Autodesk Inventor part; units mm, degrees
ref_plane "YZ Plane" through (0, 0, 0) normal (1, 0, 0) x (0, 1, 0)
ref_plane "XZ Plane" through (0, 0, 0) normal (0, 1, 0) x (-1, 0, 0)
ref_plane "XY Plane" through (0, 0, 0) normal (0, 0, 1) x (1, 0, 0)
sketch "Sketch1" plane through (0, 0, 0) normal (0, 0, 1) x (1, 0, 0)
  line L0 (5.6444, -5.6444) -> (-5.6444, -5.6444)
  line L1 (-5.6444, -5.6444) -> (-5.6444, 5.6444)
  line L2 (-5.6444, 5.6444) -> (5.6444, 5.6444)
  line L3 (5.6444, 5.6444) -> (5.6444, -5.6444)
  point P0 (0, 0)
  point P1 (0, 0)
  dimension "d0" = 11.2889
extrude "Extrusion1" add sketch "Sketch1" along normal blind 8.4667
ref_plane "Work Plane1" through (0, 5.6444, 8.4667) normal (-1, 0, 0) x (0, -1, 0)
sketch "Sketch2" plane through (0, 5.6444, 8.4667) normal (-1, 0, 0) x (0, -1, 0)
  line L0 (5.6444, -8.4667) -> (-7.0556, -8.4667)
  line L1 (0, -8.4667) -> (11.2889, -8.4667)
  line L2 (5.6444, -8.4667) -> (5.6444, -14.8167)
  arc A0 (-7.0556, -8.4667) -> (5.6444, -14.8167) centre (5.6444, 1.0583) ccw
  dimension "d3" = 12.7
  dimension "d4" = 6.35
revolve "Revolution1" add sketch "Sketch2" angle 360 about axis through (0, 0, 0) along (0, 0, -1)
properties part number "Driver Shaft Cap"
Geometry: final body of the model. Coordinates: model frame, mm. A direction names the side the tool comes from. Coordinates: 2 decimals unless noted, no trailing zeros. Loops run counter-clockwise (first coordinate to the right, second up) from the corner with the lowest first, then second, coordinate; pieces in that order, holes last. Notation, with made-up numbers: (9, 35) - (68, 35) arc R34 cw to (68, 68) - close; hole circle Ø11 at (-30.5, 48.5). An arc over 180 degrees is marked (long way). Put each result on its own line as item: value. Start each with the question number.
Q1. Set-up query: faces 1 (the flat face through (5.644, 0, 4)), 2 (the flat face through (0, 5.644, 4)), 3 (the flat face through (0, 0, 8.467)), 4 (the flat face through (-5.644, 0, 4)), 5 (the flat face through (0, -5.644, 4)). Return all of +Z, -Z, +X, -X, +Y, -Y with unobstructed straight access to the full face (end or side cutting, diameter ignored); none if empty.
Q2. Pin query (flat end, axial travel): pin 1 Ø4 at (x, y) = (3.5, -3) entering from -Z; pin 2 Ø3 at (y, z) = (1, -3) entering from +X; pin 3 Ø8 at (x, z) = (4, 3) entering from +Y; pin 4 Ø7.5 at (x, y) = (3.5, 6) entering from +Z. Return the tip coordinate at first contact, or that it passes through.
Q3. Cut plane C-C, the plane z = 4.25. Return loops of the section in (x, y).
Q4. Line query: line 1 (X direction, y = 3.75, z = 7.75); line 2 (Z direction, x = -6, y = -6.75). Output: solid intervals per line, ascending.
Q5. Cut plane D-D, the plane x = -8.75. Return loops of the section in (y, z) (3 decimals), and give its area (3 significant figures).
Q6. Cut plane A-A, the plane x = 4.75. Return loops of the section in (y, z) (3 decimals).
Filled sheet:
1. face 1: +Z, +X, +Y, -Y
1. face 2: +Z, +X, -X, +Y
1. face 3: +Z, +X, -X, +Y, -Y
1. face 4: +Z, -X, +Y, -Y
1. face 5: +Z, +X, -X, -Y
2. pin 1: z = -6.13
2. pin 2: x = 11.38
2. pin 3: y = 12.63
2. pin 4: z = 8.47
3. outline: (-5.64, -5.64) - (5.64, -5.64) - (5.64, 5.64) - (-5.64, 5.64) - close
4. line 1: -5.64 to 5.64
4. line 2: -3.53 to 0
5. outline: (-9.205, 0) arc R13.246 ccw to (9.205, 0) - close
5. area: 47.1 mm²
6. outline: (-11.778, 0) arc R15.148 ccw to (11.778, 0) - (5.644, 0) - (5.644, 8.467) - (-5.644, 8.467) - (-5.644, 0) - close
